from build123d import *

# Parameters (mm, degrees)
F1_DEPTH = 260
F3_DEPTH = 60.001
F4_R     = 4.5
F5_DEPTH = 60.001


with BuildPart() as f1:
    # F0 (on Front) → F1 (new body)
    with BuildSketch(Plane.XZ):
        Polygon((60, 0), (0, 0), (0, -60), (2.5, -60), (2.5, -2.5), (60, -2.5), align=None)
    extrude(amount=F1_DEPTH)

    # F2 (on face) → F3 (cut, through all)
    with BuildSketch(Plane(origin=(0, 0, 0), x_dir=(0, -1, 0), z_dir=(-1, 0, 0))):
        Polygon((0, 0), (0, -60), (60, 0), align=None)
        Polygon((260, -60), (260, 0), (200, -60), align=None)
    extrude(amount=-F3_DEPTH, mode=Mode.SUBTRACT)

    # F4 (on face) → F5 (cut, through all)
    with BuildSketch(Plane.XY):
        with Locations((30, -110)):
            Circle(F4_R)
        with Locations((30, -210)):
            Circle(F4_R)
    extrude(amount=-F5_DEPTH, mode=Mode.SUBTRACT)


solid = f1.part
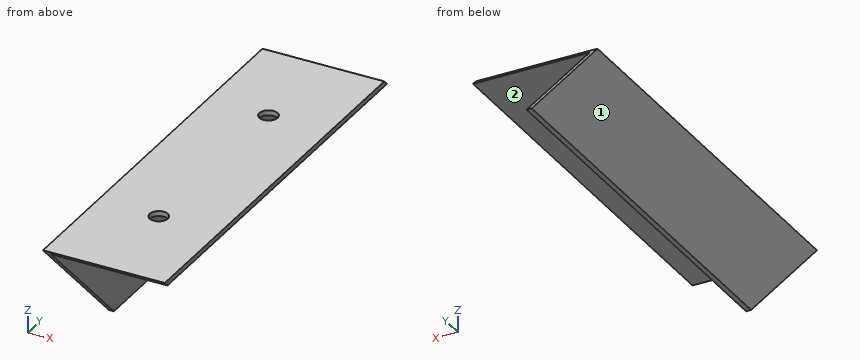
Geometry check sheet. Reference: the model listing, model coordinates, mm. Face numbers are marked on the shaded views. A direction names the side the tool comes from. Give positions to 0.01 mm unless a question says otherwise; leave off trailing zeros. Order: outer loops, then holes, each group sorted by start corner. A loop starts at its lowest first (then second) coordinate and runs counter-clockwise, first axis right, second up.
1) Cross-section at C-C (y = -110). Record the boundary of the cut face in (x, z), then the cut area to 3 significant figures.
Results are:
outline: (0, -60) - (2.5, -60) - (2.5, -2.5) - (25.5, -2.5) - (25.5, 0) - (0, 0) - close; (34.5, -2.5) - (60, -2.5) - (60, 0) - (34.5, 0) - close
area: 271 mm2
2) Material ranges on probe 1 along Y at (x, z) = (30, -1); probe 2 along Y at (x, z) = (30, -1.85); probe 3 along Z at (x, y) = (46, -72), recorded low to high.
Results are:
probe 1: y = -259 to -214.5, -205.5 to -114.5, -105.5 to -59
probe 2: y = -258.15 to -214.5, -205.5 to -114.5, -105.5 to -58.15
probe 3: z = -2.5 to 0
3) Cross-section at B-B (x = 30). Record the boundary of the cut face in (y, z).
Results are:
outline: (-260, 0) - (-257.5, -2.5) - (-214.5, -2.5) - (-214.5, 0) - close; (-205.5, -2.5) - (-114.5, -2.5) - (-114.5, 0) - (-205.5, 0) - close; (-105.5, -2.5) - (-57.5, -2.5) - (-60, 0) - (-105.5, 0) - close
4) Cross-section at A-A (y = -210). Record the boundary of the cut face in (x, z), then the cut area to 3 significant figures.
Results are:
outline: (0, -50) - (2.5, -50) - (2.5, -2.5) - (25.5, -2.5) - (25.5, 0) - (0, 0) - close; (34.5, -2.5) - (60, -2.5) - (60, 0) - (34.5, 0) - close
area: 246 mm2
5) Tool access check on the marked faces 1 and 2. Record the directions out of +Z, -Z, +X, -X, +Y, -Y that give a thin tool (end or side, any length) a straight path to the whole face; none if there is none.
Results are:
face 1: +Z, -Z, -X, +Y, -Y
face 2: -Z, +X, +Y, -Y
6) Cross-section at D-D (z = -24). Record the boundary of the cut face in (x, y), then the cut area to 3 significant figures.
Results are:
outline: (0, -236) - (2.5, -236) - (2.5, -36) - (0, -36) - close
area: 500 mm2
7) Gauge pin test, flat ends, axial feed: pin 1 (6 mm diameter, centred on x = 54, y = -122.5, fed in from -Z); pin 2 (2 mm diameter, centred on y = -57.5, z = -24.5, fed in from +X). Record the tip position at first contact, or that the pin passes through.
Results are:
pin 1: stops at z = -2.5
pin 2: stops at x = 2.5
